```python
from build123d import *

# Parameters (mm, degrees)
F0_W      = 1562.1
F0_H      = 662.792688
F1_DEPTH  = 12.7
F2_W      = 1600.2
F2_H      = 700.892688
F2_W_2    = 1562.1
F2_H_2    = 662.792688
F3_DEPTH  = 25.4
F5_DEPTH  = 0.0254
F7_DEPTH  = 0.0508
F8_W      = 88.9
F8_H      = 1123.95
F9_DEPTH  = 34.925
F10_R     = 3.175
F11_DEPTH = 60.326
F12_R     = 12.7
F13_DEPTH = 12.7


with BuildPart() as f1:
    # F0 (on Front) → F1 (new body)
    with BuildSketch(Plane.XZ):
        Rectangle(F0_W, F0_H)
    extrude(amount=F1_DEPTH)

    # F2 (on Front) → F3 (join)
    with BuildSketch(Plane.XZ):
        Rectangle(F2_W, F2_H)
        Rectangle(F2_W_2, F2_H_2, mode=Mode.SUBTRACT)
    extrude(amount=F3_DEPTH)

    # F4 (on face) → F5 (join)
    with BuildSketch(Plane.XZ.offset(12.7)):
        Polygon((-118.156804, 0), (0, 0), (-538.677069, 331.396344), (-656.833873, 331.396344), align=None)
        Polygon((-242.372931, 0), (-781.05, 331.396344), (-781.05, 258.705793), (-360.529735, 0), align=None)
        Polygon((-596.843343, 0), (-478.686539, 0), (-781.05, 186.015242), (-781.05, 113.324691), align=None)
        Polygon((-781.05, 0), (-715.000147, 0), (-781.05, 40.63414), align=None)
        Polygon((-420.520265, 331.396344), (0, 72.690551), (0, 145.381102), (-302.363461, 331.396344), align=None)
        Polygon((-184.206657, 331.396344), (0, 218.071652), (0, 290.762203), (-66.049853, 331.396344), align=None)
    extrude(amount=F5_DEPTH)

    # F6 (on face) → F7 (join)
    with BuildSketch(Plane.XZ.offset(12.7)):
        Polygon((-596.843343, 0), (-781.05, 113.324691), (-781.05, 40.63414), (-715.000147, 0), align=None)
        Polygon((-781.05, 258.705793), (-781.05, 186.015242), (-478.686539, 0), (-360.529735, 0), align=None)
        Polygon((-656.833873, 331.396344), (-781.05, 331.396344), (-242.372931, 0), (-118.156804, 0), align=None)
        Polygon((-420.520265, 331.396344), (-538.677069, 331.396344), (0, 0), (0, 72.690551), align=None)
        Polygon((-184.206657, 331.396344), (-302.363461, 331.396344), (0, 145.381102), (0, 218.071652), align=None)
        Polygon((0, 331.396344), (-66.049853, 331.396344), (0, 290.762203), align=None)
    extrude(amount=F7_DEPTH)

    # F8 (on Front) → F9 (join)
    with BuildSketch(Plane.XZ):
        with Locations((736.6, -255.978656)):
            Rectangle(F8_W, F8_H)
        with Locations((-736.6, -255.978656)):
            Rectangle(F8_W, F8_H)
    extrude(amount=-F9_DEPTH)

    # F10 (on face) → F11 (cut, through all)
    with BuildSketch(Plane(origin=(0, 34.925, 0), x_dir=(-1, 0, 0), z_dir=(0, 1, 0))):
        with Locations((-750.8875, -687.778656)):
            Circle(F10_R)
        with Locations((-750.8875, -560.778656)):
            Circle(F10_R)
        with Locations((750.8875, -560.778656)):
            Circle(F10_R)
        with Locations((750.8875, -687.778656)):
            Circle(F10_R)
    extrude(amount=-F11_DEPTH, mode=Mode.SUBTRACT)

    # F12 (on face) → F13 (cut)
    with BuildSketch(Plane(origin=(0, 34.925, 0), x_dir=(-1, 0, 0), z_dir=(0, 1, 0))):
        with Locations((-750.8875, -687.778656)):
            Circle(F12_R)
        with Locations((-750.8875, -560.778656)):
            Circle(F12_R)
        with Locations((750.8875, -687.778656)):
            Circle(F12_R)
        with Locations((750.8875, -560.778656)):
            Circle(F12_R)
    extrude(amount=-F13_DEPTH, mode=Mode.SUBTRACT)


solid = f1.part
```
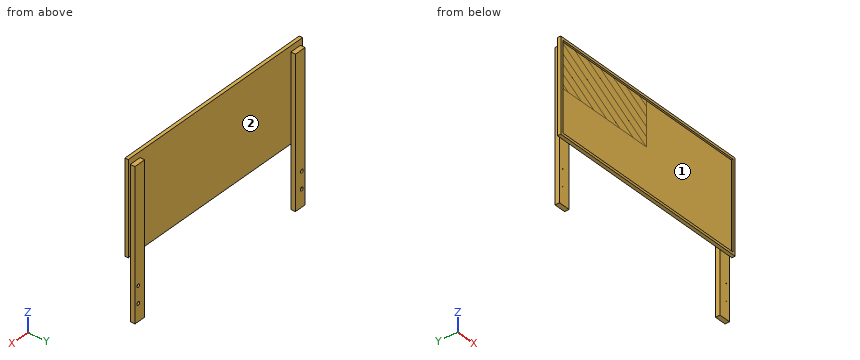
Design review of the part built by this model. Coordinates are the model's own, in mm. Face numbers are marked on the shaded views. Coordinates: 2 decimals unless noted, no trailing zeros. Loops run counter-clockwise (first coordinate to the right, second up) from the corner with the lowest first, then second, coordinate; pieces in that order, holes last. Notation, with made-up numbers: (-34.5, 39.5) - (-10.5, 39.5) arc R17 ccw to (-10.5, 46.5) - close; hole circle Ø4 at (-25, 7). An arc over 180 degrees is marked (long way). Use CSV: the item, a comma, the result in double quotes. Start each with the question number.
1) Consider section C-C on z = -212.5. Write out the cut boundary in (x, y) (3 decimals), then the cut area to 3 significant figures.
2) Wall thickness on L1, parallel to X at y = -13.5, z = -100.5; L2, parallel to X at y = 21, z = 82.5; L3, parallel to Z at x = -33, y = -13.5: over which ranges is each line inside the solid? List them lowest first. Write a range as from..to.
3) The part is to be moulded in two halves that separate along X. For the marked faces 1 and 2, say which applies: +X half, -X half, draft (parallel to the pull), parting line (faces both ways), or undercut.
4) For pin 1 Ø17.5 at (x, y) = (-723, 24) entering from +Z; pin 2 Ø10.5 at (y, z) = (13, -186.5) entering from -X; pin 3 Ø1.5 at (x, z) = (215, 104.5) entering from -Y, all flat-tipped, find the tip position at first contact; note any pin that passes through.
5) Consider section B-B on x = 136. Write out the cut boundary in (y, z).
6) Consider section A-A on z = -601. Write out the cut boundary in (x, y) (3 decimals).
Geometry says:
1,outline,"(-800.1, -25.4) - (-781.05, -25.4) - (-781.05, -12.7) - (781.05, -12.7) - (781.05, -25.4) - (800.1, -25.4) - (800.1, 0) - (781.05, 0) - (781.05, 34.925) - (692.15, 34.925) - (692.15, 0) - (-692.15, 0) - (-692.15, 34.925) - (-781.05, 34.925) - (-781.05, 0) - (-800.1, 0) - close"
1,area,"27,000 mm^2"
2,L1,"-800.1..-781.05, 781.05..800.1"
2,L2,"-781.05..-692.15, 692.15..781.05"
2,L3,"-350.45..-331.4, 331.4..350.45"
3,face 1,"undercut"
3,face 2,"undercut"
4,pin 1,"z = 306"
4,pin 2,"x = -781.05"
4,pin 3,"y = -12.7"
5,outline,"(-25.4, -350.45) - (0, -350.45) - (0, 350.45) - (-25.4, 350.45) - (-25.4, 331.4) - (-12.7, 331.4) - (-12.7, -331.4) - (-25.4, -331.4) - close"
6,outline,"(-781.05, 0) - (-692.15, 0) - (-692.15, 34.925) - (-781.05, 34.925) - close; (692.15, 0) - (781.05, 0) - (781.05, 34.925) - (692.15, 34.925) - close"
